from build123d import *

# Parameters (mm, degrees)
F1_DEPTH  = 12.7
F3_DEPTH  = 25.4
F6_DEPTH  = 25.4
F9_DEPTH  = 25.4
F11_DEPTH = 1.778
F12_DEPTH = 1.016
F13_DEPTH = 1.016


with BuildPart() as f1:
    # F0 (on Front) → F1 (new body, symmetric)
    with BuildSketch(Plane.XZ):
        with BuildLine():
            Line((-12.7, 0), (0, 0))
            Line((0, 0), (12.7, 0))
            ThreePointArc((12.7, 0), (15.24, 2.54), (12.7, 5.08))
            Line((12.7, 5.08), (-12.7, 5.08))
            ThreePointArc((-12.7, 5.08), (-15.24, 2.54), (-12.7, 0))
        make_face()
    extrude(amount=F1_DEPTH, both=True)

    # F2 (on Right) → F3 (cut, symmetric)
    with BuildSketch(Plane.YZ):
        with BuildLine():
            ThreePointArc((10.16, 5.08), (12.7, 2.54), (10.16, 0))
            Line((10.16, 0), (29.21, 0))
            Line((29.21, 0), (29.21, 5.08))
            Line((29.21, 5.08), (10.16, 5.08))
        make_face()
        with BuildLine():
            ThreePointArc((-10.16, 0), (-12.7, 2.54), (-10.16, 5.08))
            Line((-10.16, 5.08), (-29.21, 5.08))
            Line((-29.21, 5.08), (-29.21, 0))
            Line((-29.21, 0), (-10.16, 0))
        make_face()
    extrude(amount=F3_DEPTH, both=True, mode=Mode.SUBTRACT)

    # F5 (on line) → F6 (cut, symmetric)
    with BuildSketch(Plane(origin=(0, 0, 0), x_dir=(-0.8660254038, -0.5, 0), z_dir=(-0.5, 0.8660254038, 0))):
        with BuildLine():
            ThreePointArc((10.16, 5.08), (12.7, 2.54), (10.16, 0))
            Line((10.16, 0), (29.21, 0))
            Line((29.21, 0), (29.21, 5.08))
            Line((29.21, 5.08), (10.16, 5.08))
        make_face()
        with BuildLine():
            ThreePointArc((-10.16, 0), (-12.7, 2.54), (-10.16, 5.08))
            Line((-10.16, 5.08), (-29.21, 5.08))
            Line((-29.21, 5.08), (-29.21, 0))
            Line((-29.21, 0), (-10.16, 0))
        make_face()
    extrude(amount=F6_DEPTH, both=True, mode=Mode.SUBTRACT)

    # F8 (on line) → F9 (cut, symmetric)
    with BuildSketch(Plane(origin=(0, 0, 0), x_dir=(-0.8660254038, 0.5, 0), z_dir=(0.5, 0.8660254038, 0))):
        with BuildLine():
            ThreePointArc((10.16, 5.08), (12.7, 2.54), (10.16, 0))
            Line((10.16, 0), (29.21, 0))
            Line((29.21, 0), (29.21, 5.08))
            Line((29.21, 5.08), (10.16, 5.08))
        make_face()
        with BuildLine():
            ThreePointArc((-10.16, 0), (-12.7, 2.54), (-10.16, 5.08))
            Line((-10.16, 5.08), (-29.21, 5.08))
            Line((-29.21, 5.08), (-29.21, 0))
            Line((-29.21, 0), (-10.16, 0))
        make_face()
    extrude(amount=F9_DEPTH, both=True, mode=Mode.SUBTRACT)

    # F10 (on face) → F11 (join)
    with BuildSketch(Plane.XY.offset(5.08)):
        Polygon((-5.230878735, 9.0601477372), (-5.865878735, 10.16), (-11.7317574699, 0), (-5.865878735, -10.16), (-5.230878735, -9.0601477372), (-10.4617574699, 0), align=None)
        Polygon((-11.7317574699, 0), (-5.865878735, 10.16), (-6.500878735, 11.2598522628), (-13.0017574699, 0), (-6.500878735, -11.2598522628), (-5.865878735, -10.16), align=None)
        Polygon((11.7317574699, 0), (5.865878735, 10.16), (5.230878735, 9.0601477372), (10.4617574699, 0), (5.230878735, -9.0601477372), (5.865878735, -10.16), align=None)
        Polygon((6.500878735, 11.2598522628), (5.865878735, 10.16), (11.7317574699, 0), (5.865878735, -10.16), (6.500878735, -11.2598522628), (13.0017574699, 0), align=None)
    extrude(amount=F11_DEPTH)

    # F10 (on face) → F12 (cut)
    with BuildSketch(Plane.XY.offset(5.08)):
        Polygon((6.500878735, 11.2598522628), (5.865878735, 10.16), (11.7317574699, 0), (5.865878735, -10.16), (6.500878735, -11.2598522628), (13.0017574699, 0), align=None)
        Polygon((-11.7317574699, 0), (-5.865878735, 10.16), (-6.500878735, 11.2598522628), (-13.0017574699, 0), (-6.500878735, -11.2598522628), (-5.865878735, -10.16), align=None)
    extrude(amount=F12_DEPTH, mode=Mode.SUBTRACT)

    # F10 (on face) → F13 (join)
    with BuildSketch(Plane.XY.offset(5.08)):
        Polygon((10.4617574699, 0), (5.230878735, 9.0601477372), (-5.230878735, 9.0601477372), (-10.4617574699, 0), (-5.230878735, -9.0601477372), (5.230878735, -9.0601477372), align=None)
    extrude(amount=F13_DEPTH)


solid = f1.part
For this review, take the finished solid that the model builds, in its own axes (mm). A direction names the side the tool comes from. Give positions to 0.01 mm unless a question says otherwise; leave off trailing zeros. Order: outer loops, then holes, each group sorted by start corner. A loop starts at its lowest first (then second) coordinate and runs counter-clockwise, first axis right, second up. Notation, with made-up numbers: M 19.25,16.5 L 45.25,16.5 A32 ccw 45.25,44.5 Z; hole C -31,-13.5 d3. An arc over 180 degrees is marked long. Answer in a Markdown table with one row per item. Add a question column.
(1) Consider section B-B on z = 2.54. State the section outline as (x, y) points, and give its area (3 significant figures).
(2) Mouldability with a two-part tool opening along Y and no side actions: class faces 1 (the face through (0.1, 9.06, 5.6)), 2 (the face through (-5.734, -9.931, 6.154)), 3 (the face through (-7.88, 4.47, 6.47)) as +Y half, -Y half, draft (parallel to the pull), parting line (faces both ways), or undercut.
(3) For pin 1 (0.5 mm diameter, centred on x = 0, y = 9.5, fed in from +Z); pin 2 (9 mm diameter, centred on x = 2, y = -0.5, fed in from +Z); pin 3 (3.5 mm diameter, centred on x = 11, y = 5.5, fed in from -Z), all flat-tipped, find the tip position at first contact; note any pin that passes through.
(4) Wall thickness on probe 1 along Z at (x, y) = (-3, 9.5); probe 2 along Y at (x, z) = (-8, 6.75); probe 3 along Z at (x, y) = (5.25, -1): over which ranges is each line inside the solid? List them lowest first. Write a range as [from, to].
(5) Consider section A-A on x = 4.25. State the section outline as (y, z) points, and give its area (3 significant figures).
(6) For faces 4 (the face through (8.84, -5.01, 5.58)), 5 (the face through (5.734, 9.931, 6.154)), 6 (the face through (9.706, -5.709, 6.472)), 7 (the face through (-7.81, -4.59, 6.47)), list the 3-axis set-ups (+Z, -Z, +X, -X, +Y, -Y) from which the entire face can be reached by the end or side of a thin tool; tool diameter is ignored.
(7) Consider section C-C on z = 0.5. State the section outline as (x, y) points, and give its area (3 significant figures).
Evaluation:
| question | item | result |
|---|---|---|
| 1 | outline | M -14.66,0 L -7.33,-12.7 L 7.33,-12.7 L 14.66,0 L 7.33,12.7 L -7.33,12.7 Z |
| 1 | area | 559 mm^2 |
| 2 | face 1 | +Y half |
| 2 | face 2 | -Y half |
| 2 | face 3 | undercut |
| 3 | pin 1 | stops at z = 5.08 |
| 3 | pin 2 | stops at z = 6.1 |
| 3 | pin 3 | stops at z = 0.03 |
| 4 | probe 1 | z = [0, 5.08] |
| 4 | probe 2 | y = [-8.66, -4.26], [4.26, 8.66] |
| 4 | probe 3 | z = [0, 6.1] |
| 5 | outline | M -10.16,0 L 10.16,0 A2.54 ccw 10.16,5.08 L 9.06,5.08 L 9.06,6.1 L -9.06,6.1 L -9.06,5.08 L -10.16,5.08 A2.54 ccw Z |
| 5 | area | 142 mm^2 |
| 6 | face 4 | +X, -Y |
| 6 | face 5 | +Z, +Y |
| 6 | face 6 | +Z, +X, -Y |
| 6 | face 7 | +Z |
| 7 | outline | M -13.48,0 L -6.74,-11.67 L 6.74,-11.67 L 13.48,0 L 6.74,11.67 L -6.74,11.67 Z |
| 7 | area | 472 mm^2 |
